Check sheet for the modelled part. Datum: model origin and axes. Units: mm. Face numbers are marked on the shaded views. A direction names the side the tool comes from. Give positions to 0.01 mm unless a question says otherwise; leave off trailing zeros. Order: outer loops, then holes, each group sorted by start corner. A loop starts at its lowest first (then second) coordinate and runs counter-clockwise, first axis right, second up.
from build123d import *

# Parameters (mm, degrees)
SKETCH1_R          = 3.175
EXTRUDE1_DEPTH     = 45.72
CHAMFER1_SIZE      = 0.635
EXTRUDE7_DEPTH     = 37.195
SKETCH14_R         = 1.651
CUT_EXTRUDE1_DEPTH = 2.2225


with BuildPart() as part:
    # Sketch1 → Extrude1 (new body, symmetric)
    with BuildSketch(Plane.XY):
        Circle(SKETCH1_R)
    extrude(amount=EXTRUDE1_DEPTH, both=True)

    # Chamfer1
    chamfer1_edges = [part.edges().sort_by_distance(p)[0] for p in [
        (-3.175, 0, -45.72),
        (-3.175, 0, 45.72),
    ]]
    chamfer(chamfer1_edges, length=CHAMFER1_SIZE)

    # Sketch13 → Extrude7 (cut, through all)
    with BuildSketch(Plane.XY.offset(9.525)):
        with BuildLine():
            Line((-2.909935566, 1.27), (2.909935566, 1.27))
            ThreePointArc((2.909935566, 1.27), (0, 3.175), (-2.909935566, 1.27))
        make_face()
    extrude(amount=EXTRUDE7_DEPTH, mode=Mode.SUBTRACT)

    # Sketch14 → Cut-Extrude1 (cut)
    with BuildSketch(Plane(origin=(0, 1.27, 0), x_dir=(1, 0, 0), z_dir=(0, 1, 0))):
        with Locations((0, -40.386)):
            Circle(SKETCH14_R)
    extrude(amount=-CUT_EXTRUDE1_DEPTH, mode=Mode.SUBTRACT)


solid = part.part
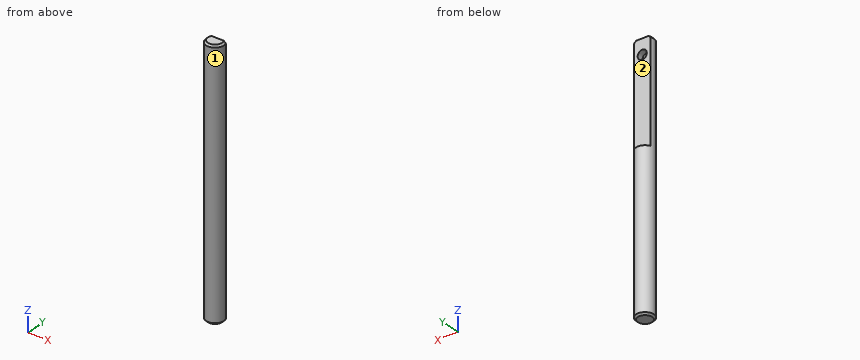
1) Section check C-C, the plane z = 2. Record the cut outline in (x, y) (3 decimals).
Recorded:
outline: circle Ø6.35 at (0, 0)
2) Section check B-B, the plane y = 0. Record the cut outline in (x, z) (3 decimals), then the cut area to 3 significant figures.
Recorded:
outline: (-3.175, -45.085) - (-2.54, -45.72) - (2.54, -45.72) - (3.175, -45.085) - (3.175, 45.085) - (2.54, 45.72) - (-2.54, 45.72) - (-3.175, 45.085) - close; hole circle Ø3.302 at (0, 40.386)
area: 571 mm2
3) Material ranges on L1, parallel to Z at x = 0, y = 0.6 (3 decimals); L2, parallel to Y at x = 0, z = 17 (3 decimals); L3, parallel to Z at x = -1, y = -0.5, recorded low to high.
Recorded:
L1: z = -45.72 to 38.735, 42.037 to 45.72
L2: y = -3.175 to 1.27
L3: z = -45.72 to 39.07, 41.7 to 45.72
4) Set-up check for the marked faces 1 and 2: record each of +Z, -Z, +X, -X, +Y, -Y from which the full face is reachable in a straight line by a thin tool's end or side.
Recorded:
face 1: +Z, -Z
face 2: +Z, +X, -X, +Y
5) Section check A-A, the plane x = 0. Record the cut outline in (y, z) (1 decimal), then the cut area to 3 significant figures.
Recorded:
outline: (-3.2, -45.1) - (-2.5, -45.7) - (2.5, -45.7) - (3.2, -45.1) - (3.2, 9.5) - (1.3, 9.5) - (1.3, 38.7) - (-1, 38.7) - (-1, 42) - (1.3, 42) - (1.3, 45.7) - (-2.5, 45.7) - (-3.2, 45.1) - close
area: 504 mm2
6) Depth check by flat-ended pin: pin 1 Ø1 at (y, z) = (-2.5, -33) entering from +X; pin 2 Ø1.5 at (y, z) = (2, -23.5) entering from +X; pin 3 Ø1 at (x, z) = (0, 40) entering from +Y. Enter the tip coordinate at first touch or a pass-through.
Recorded:
pin 1: stops at x = 2.47
pin 2: stops at x = 2.92
pin 3: stops at y = -0.95
